The drawing under review shows one solid part. Ordinate dimensions are in mm from its lowest x, y, z. A direction names the side the tool comes from. Round coordinates to 2 decimals unless told otherwise and drop trailing zeros. Order: outer loops, then holes, each group sorted by start corner. A loop starts at its lowest first (then second) coordinate and runs counter-clockwise, first axis right, second up. Notation, with made-up numbers: M 6.25,-26.5 L 17.25,-26.5 A24 ccw 17.25,4.5 Z; hole C -16.5,-25.5 d2. An arc over 180 degrees is marked long. Answer as a JSON object with one key per item and string values.
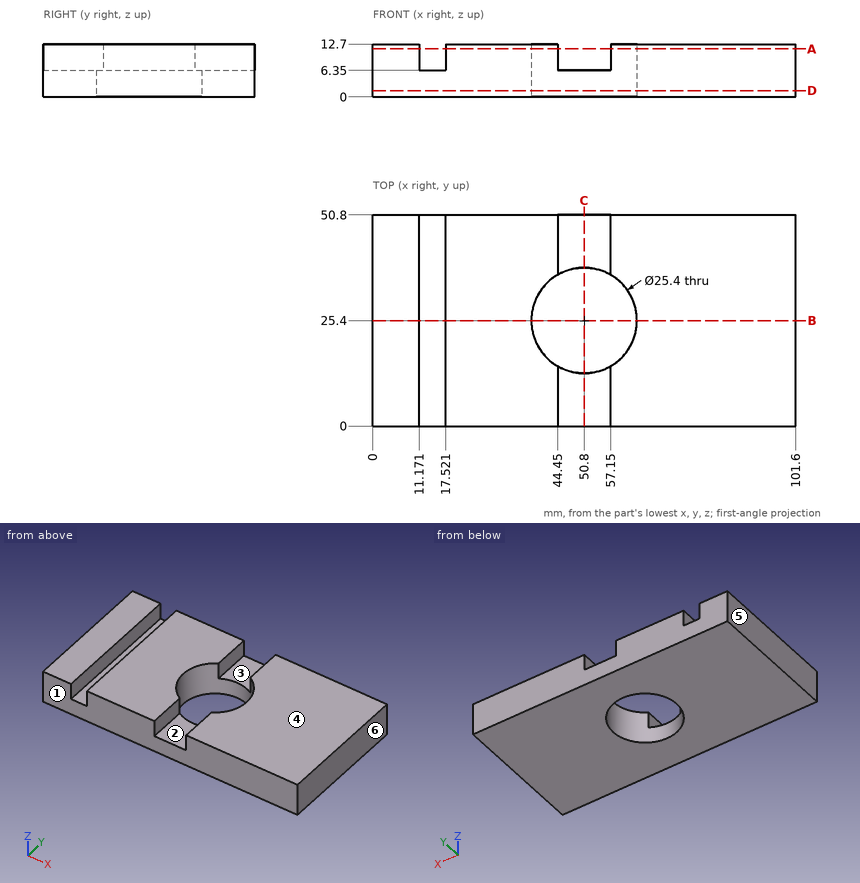
1) Machinability: for the marked faces 1 and 2, which of the approach directions +Z, -Z, +X, -X, +Y, -Y give a long, thin tool a straight path to every point of the face, cutting with its end or side? Answer none if there is none.
Geometry check:
{"face 1": "+Z, -Z, +X, -X, -Y", "face 2": "+Z, +Y, -Y"}
2) Add section B-B on y = 25.4. State the section outline as (x, z) points.
Geometry check:
{"outline": "M 0,0 L 38.1,0 L 38.1,12.7 L 17.52,12.7 L 17.52,6.35 L 11.17,6.35 L 11.17,12.7 L 0,12.7 Z; M 63.5,0 L 101.6,0 L 101.6,12.7 L 63.5,12.7 Z"}
3) Add section C-C on x = 50.8. State the section outline as (y, z) points, and give its area (3 significant figures).
Geometry check:
{"outline": "M 0,0 L 12.7,0 L 12.7,6.35 L 0,6.35 Z; M 38.1,0 L 50.8,0 L 50.8,6.35 L 38.1,6.35 Z", "area": "161 mm²"}
4) Mouldability with a two-part tool opening along X and no side actions: class the marked faces 3, 4, 5 and 6 as +X half, -X half, draft (parallel to the pull), parting line (faces both ways), or undercut.
Geometry check:
{"face 3": "undercut", "face 4": "draft", "face 5": "-X half", "face 6": "+X half"}
5) Add section D-D on z = 1.5. State the section outline as (x, y) points.
Geometry check:
{"outline": "M 0,0 L 101.6,0 L 101.6,50.8 L 0,50.8 Z; hole C 50.8,25.4 d25.4"}
6) Insertion check: P1, Ø10, axis at x = 49.5, y = 5, coming from the +Z side. The pin has a flat end and moves straight along its axis. Give the tip position at first contact, or say it passes through.
Geometry check:
{"P1": "stops at z = 6.35"}
7) For L1, parallel to X at y = 4.5, z = 7; L2, parallel to Y at x = 50.8, z = 4.25; L3, parallel to X at y = 25.4, z = 5.25, list the stretches that pass through material, from the lowest coordinate up.
Geometry check:
{"L1": "x = 0 to 11.17, 17.52 to 44.45, 57.15 to 101.6", "L2": "y = 0 to 12.7, 38.1 to 50.8", "L3": "x = 0 to 38.1, 63.5 to 101.6"}
8) Add section A-A on z = 11.5. State the section outline as (x, y) points, and give its area (3 significant figures).
Geometry check:
{"outline": "M 0,0 L 11.17,0 L 11.17,50.8 L 0,50.8 Z; M 17.52,0 L 44.45,0 L 44.45,14.4 A12.7 cw 44.45,36.4 L 44.45,50.8 L 17.52,50.8 Z; M 57.15,0 L 101.6,0 L 101.6,50.8 L 57.15,50.8 L 57.15,36.4 A12.7 cw 57.15,14.4 Z", "area": "4,000 mm²"}
